Could you check a few things on this model? Use its own coordinates, in mm. A direction names the side the tool comes from. Give positions to 0.01 mm unless a question says otherwise; leave off trailing zeros. Order: outer loops, then holes, each group sorted by start corner. A loop starts at its lowest first (then second) coordinate and runs counter-clockwise, first axis right, second up.
(1) Will these pins go through, and if not, where does the flat tip stop? pin 1 (6 mm diameter, centred on x = -11, y = -15, fed in from -Z); pin 2 (10 mm diameter, centred on y = 1.5, z = -11.5, fed in from +X); pin 3 (5 mm diameter, centred on x = -2, y = -6, fed in from -Z).
(2) If we mould it in two halves opening along Z, with no side actions, what happens to faces 1 (the flat face through (-0.1, 0, 14.2)), 2 (the cylindrical face through (3.356, 14.004, -8.068))? For each: released by +Z, released by -Z, zero draft, split by the parting line, or undercut.
(3) If I drill on probe 1 along Z at (x, y) = (0, -5); probe 2 along Z at (x, y) = (0, 3); probe 3 along Y at (x, z) = (0.5, 14), over which ranges is the centre line in solid material (lowest first)?
(4) Imagine slicing it at B-B, the plane z = 0. Write out the boundary of the cut face in (x, y), then the cut area to 3 significant figures.
(5) On a 3-axis mill with a long thin cutter (end or side, diameter ignored), from which of +Z, -Z, +X, -X, +Y, -Y can I reach the whole of each face in a straight line? I mean faces 3 (the flat face through (6.34, 6.35, -14.04)), 4 (the flat face through (11.23, 0.305, -3.7)), 5 (the flat face through (-3, 17.323, -10)), 6 (the cylindrical face through (-11.646, 14.004, -0.029)). Say none if no direction works.
(6) Imagine slicing it at D-D, the plane y = -20. Write out the boundary of the cut face in (x, z).
(7) Imagine slicing it at A-A, the plane x = 0. Write out the boundary of the cut face in (y, z).
from build123d import *

# Parameters (mm, degrees)
F0_R      = 17.3355
F1_DEPTH  = 6.35
F2_R      = 14.986
F3_DEPTH  = 31.4452
F4_R      = 15.24
F5_DEPTH  = 10.9728
F6_W      = 4.1148
F6_H      = 1.09728
F8_R      = 11.6459
F9_DEPTH  = 31.75
F10_R     = 12.7
F11_DEPTH = 10.287
F13_DEPTH = 6.731


with BuildPart() as f1:
    # F0 (on Front) → F1 (new body)
    with BuildSketch(Plane.XZ):
        Circle(F0_R)
    extrude(amount=-F1_DEPTH)

    # F2 (on face) → F3 (join)
    with BuildSketch(Plane.XZ):
        Circle(F2_R)
    extrude(amount=F3_DEPTH)

    # F4 (on face) → F5 (join)
    with BuildSketch(Plane(origin=(0, 6.35, 0), x_dir=(-1, 0, 0), z_dir=(0, 1, 0))):
        Circle(F4_R)
    extrude(amount=F5_DEPTH)

    # F6 (on Right) → F7 (revolve, cut)
    with BuildSketch(Plane.YZ):
        with Locations((-2.0574, 14.43736)):
            Rectangle(F6_W, F6_H)
    revolve(axis=Axis((0, -0.221021, 0), (0, 1, 0)), mode=Mode.SUBTRACT)

    # F8 (on face) → F9 (cut)
    with BuildSketch(Plane.XZ.offset(31.4452)):
        Circle(F8_R)
    extrude(amount=-F9_DEPTH, mode=Mode.SUBTRACT)

    # F10 (on face) → F11 (cut)
    with BuildSketch(Plane.XZ.offset(-0.3048)):
        Circle(F10_R)
    extrude(amount=-F11_DEPTH, mode=Mode.SUBTRACT)

    # F12 (on face) → F13 (cut, through all)
    with BuildSketch(Plane(origin=(0, 17.3228, 0), x_dir=(-1, 0, 0), z_dir=(0, 1, 0))):
        with BuildLine():
            Line((-4.173907, 7.676207), (-6.65057, 9.560173))
            ThreePointArc((-6.65057, 9.560173), (-8.234895, 8.234895), (-9.560173, 6.65057))
            Line((-9.560173, 6.65057), (-7.676207, 4.173907))
            ThreePointArc((-7.676207, 4.173907), (-8.07249, 3.343735), (-8.379296, 2.4765))
            Line((-8.379296, 2.4765), (-11.462726, 2.0574))
            ThreePointArc((-11.462726, 2.0574), (-11.6459, 0), (-11.462726, -2.0574))
            Line((-11.462726, -2.0574), (-8.379296, -2.4765))
            ThreePointArc((-8.379296, -2.4765), (-8.07249, -3.343735), (-7.676207, -4.173907))
            Line((-7.676207, -4.173907), (-9.560173, -6.65057))
            ThreePointArc((-9.560173, -6.65057), (-8.234895, -8.234895), (-6.65057, -9.560173))
            Line((-6.65057, -9.560173), (-4.173907, -7.676207))
            ThreePointArc((-4.173907, -7.676207), (-3.343735, -8.07249), (-2.4765, -8.379296))
            Line((-2.4765, -8.379296), (-2.0574, -11.462726))
            ThreePointArc((-2.0574, -11.462726), (0, -11.6459), (2.0574, -11.462726))
            Line((2.0574, -11.462726), (2.4765, -8.379296))
            ThreePointArc((2.4765, -8.379296), (3.343735, -8.07249), (4.173907, -7.676207))
            Line((4.173907, -7.676207), (6.65057, -9.560173))
            ThreePointArc((6.65057, -9.560173), (8.234895, -8.234895), (9.560173, -6.65057))
            Line((9.560173, -6.65057), (7.676207, -4.173907))
            ThreePointArc((7.676207, -4.173907), (8.07249, -3.343735), (8.379296, -2.4765))
            Line((8.379296, -2.4765), (11.462726, -2.0574))
            ThreePointArc((11.462726, -2.0574), (11.6459, 0), (11.462726, 2.0574))
            Line((11.462726, 2.0574), (8.379296, 2.4765))
            ThreePointArc((8.379296, 2.4765), (8.07249, 3.343735), (7.676207, 4.173907))
            Line((7.676207, 4.173907), (9.560173, 6.65057))
            ThreePointArc((9.560173, 6.65057), (8.234895, 8.234895), (6.65057, 9.560173))
            Line((6.65057, 9.560173), (4.173907, 7.676207))
            ThreePointArc((4.173907, 7.676207), (3.343735, 8.07249), (2.4765, 8.379296))
            Line((2.4765, 8.379296), (2.0574, 11.462726))
            ThreePointArc((2.0574, 11.462726), (0, 11.6459), (-2.0574, 11.462726))
            Line((-2.0574, 11.462726), (-2.4765, 8.379296))
            ThreePointArc((-2.4765, 8.379296), (-3.343735, 8.07249), (-4.173907, 7.676207))
        make_face()
    extrude(amount=-F13_DEPTH, mode=Mode.SUBTRACT)


solid = f1.part
Answer block:
1. pin 1: stops at z = -12.67
1. pin 2: stops at x = 16.07
1. pin 3: stops at z = -14.99
2. face 1: zero draft
2. face 2: undercut
3. probe 1: z = -14.99 to -11.65, 11.65 to 14.99
3. probe 2: z = -17.34 to -12.7, 12.7 to 17.34
3. probe 3: y = -31.45 to -4.11, 0 to 17.32
4. outline: (-17.34, 0) - (-13.89, 0) - (-13.89, -4.11) - (-14.99, -4.11) - (-14.99, -31.45) - (-11.65, -31.45) - (-11.65, 0.3) - (-12.7, 0.3) - (-12.7, 10.59) - (-11.65, 10.59) - (-11.65, 17.32) - (-15.24, 17.32) - (-15.24, 6.35) - (-17.34, 6.35) - close; (11.65, -31.45) - (14.99, -31.45) - (14.99, -4.11) - (13.89, -4.11) - (13.89, 0) - (17.34, 0) - (17.34, 6.35) - (15.24, 6.35) - (15.24, 17.32) - (11.65, 17.32) - (11.65, 10.59) - (12.7, 10.59) - (12.7, 0.3) - (11.65, 0.3) - close
4. area: 330 mm2
5. face 3: +Y
5. face 4: none
5. face 5: +Z, -Z, +X, -X, +Y
5. face 6: +Y, -Y
6. outline: circle Ø29.97 at (0, 0); hole circle Ø23.29 at (0, 0)
7. outline: (-31.45, -14.99) - (-4.11, -14.99) - (-4.11, -13.89) - (0, -13.89) - (0, -17.34) - (6.35, -17.34) - (6.35, -15.24) - (17.32, -15.24) - (17.32, -11.65) - (10.59, -11.65) - (10.59, -12.7) - (0.3, -12.7) - (0.3, -11.65) - (-31.45, -11.65) - close; (-31.45, 11.65) - (0.3, 11.65) - (0.3, 12.7) - (10.59, 12.7) - (10.59, 11.65) - (17.32, 11.65) - (17.32, 15.24) - (6.35, 15.24) - (6.35, 17.34) - (0, 17.34) - (0, 13.89) - (-4.11, 13.89) - (-4.11, 14.99) - (-31.45, 14.99) - close
